Source: three-view drawing plus pictorial views. Frame: mm from the lowest corner of the part. Coordinates: 2 decimals unless noted, no trailing zeros. Write each loop counter-clockwise with the first axis right and the second up, starting at its lowest first coordinate (ties: lowest second). Pieces come first, ordered by that corner, then holes. Notation, with made-up numbers: (16, -14.75) - (53, -14.75) arc R31 cw to (53, 24.25) - close; hole circle Ø4 at (10.5, -29.5). An arc over 180 degrees is marked (long way). Put each result on its own line as item: value.
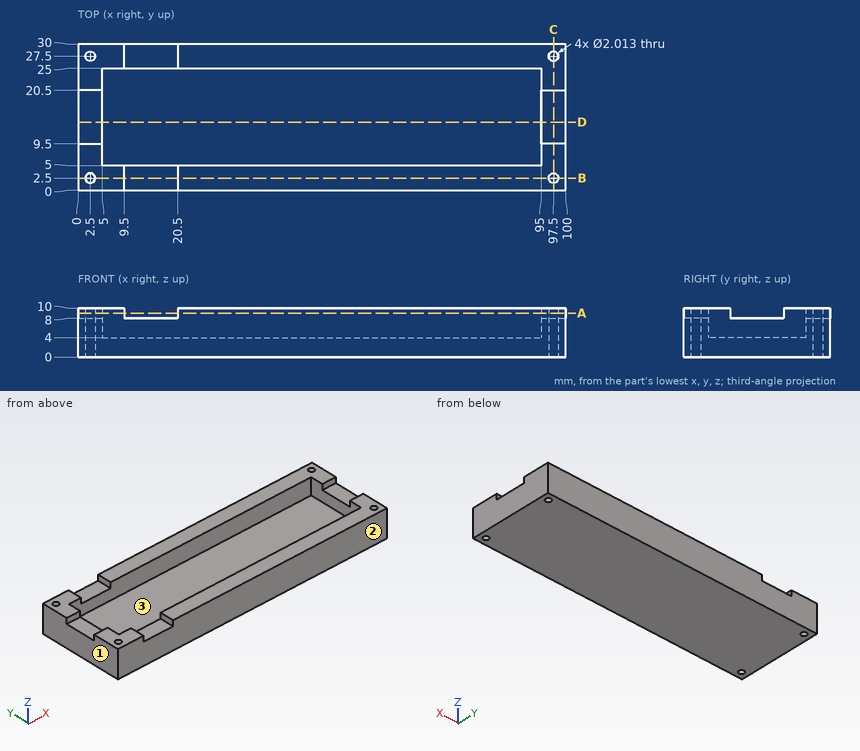
1. Section query A-A (z = 9). Return loops of the section in (x, y).
Answer below:
outline: (0, 0) - (9.5, 0) - (9.5, 5) - (5, 5) - (5, 9.5) - (0, 9.5) - close; (0, 20.5) - (5, 20.5) - (5, 25) - (9.5, 25) - (9.5, 30) - (0, 30) - close; (20.5, 0) - (100, 0) - (100, 9.5) - (95, 9.5) - (95, 5) - (20.5, 5) - close; (20.5, 25) - (95, 25) - (95, 20.5) - (100, 20.5) - (100, 30) - (20.5, 30) - close; hole circle Ø2.01 at (2.5, 2.5); hole circle Ø2.01 at (2.5, 27.5); hole circle Ø2.01 at (97.5, 2.5); hole circle Ø2.01 at (97.5, 27.5)
2. Section query B-B (y = 2.5). Return loops of the section in (x, z).
Answer below:
outline: (0, 0) - (1.49, 0) - (1.49, 10) - (0, 10) - close; (3.51, 0) - (96.49, 0) - (96.49, 10) - (20.5, 10) - (20.5, 8) - (9.5, 8) - (9.5, 10) - (3.51, 10) - close; (98.51, 0) - (100, 0) - (100, 10) - (98.51, 10) - close
3. Pin query (flat end, axial travel): pin 1 Ø10 at (x, y) = (62.5, 16) entering from +Z; pin 2 Ø1.5 at (x, y) = (12.5, 27.5) entering from +Z. Return the tip coordinate at first contact, or that it passes through.
Answer below:
pin 1: stops at z = 4
pin 2: stops at z = 8
4. Section query C-C (x = 97.5). Return loops of the section in (y, z).
Answer below:
outline: (0, 0) - (1.49, 0) - (1.49, 10) - (0, 10) - close; (3.51, 0) - (26.49, 0) - (26.49, 10) - (20.5, 10) - (20.5, 8) - (9.5, 8) - (9.5, 10) - (3.51, 10) - close; (28.51, 0) - (30, 0) - (30, 10) - (28.51, 10) - close
5. Section query D-D (y = 14). Return loops of the section in (x, z), then the cut area to 3 significant figures.
Answer below:
outline: (0, 0) - (100, 0) - (100, 8) - (95, 8) - (95, 4) - (5, 4) - (5, 8) - (0, 8) - close
area: 440 mm²
6. Ray query, probe 1 along Y at (x, z) = (97.5, 4.5); probe 2 along X at (y, z) = (27.5, 3); probe 3 along X at (y, z) = (17, 7.25). Return the intervals inside material, ascending. Write a range as from..to.
Answer below:
probe 1: y = 0..1.49, 3.51..26.49, 28.51..30
probe 2: x = 0..1.49, 3.51..96.49, 98.51..100
probe 3: x = 0..5, 95..100
7. Mould query, pull axis Y, two halves, no side actions, for the marked faces 1, 2 and 3. Classes: +Y half, -Y half, draft (parallel to the pull), parting line (faces both ways), or undercut.
Answer below:
face 1: draft
face 2: -Y half
face 3: undercut
